from build123d import *

# Parameters (mm, degrees)
F1_DEPTH = 50
F2_R     = 8.5
F3_DEPTH = 40


with BuildPart() as f1:
    # F0 (on Top) → F1 (new body)
    with BuildSketch(Plane.XY):
        Polygon((1.650066, 3.020267), (-13.349934, 3.020267), (-13.349934, -15.979733), (1.650066, -15.979733), (7.459541, -10.479733), (7.459541, -2.479733), align=None)
    extrude(amount=F1_DEPTH)

    # F2 (on Top) → F3 (cut)
    with BuildSketch(Plane.XY):
        with Locations((-2.349934, -6.479733)):
            Circle(F2_R)
    extrude(amount=F3_DEPTH, mode=Mode.SUBTRACT)


solid = f1.part
Work out the finished part from the listing and answer in its coordinate system (mm). Round coordinates to 2 decimals unless told otherwise and drop trailing zeros. Write each loop counter-clockwise with the first axis right and the second up, starting at its lowest first coordinate (ties: lowest second). Pieces come first, ordered by that corner, then holes. Notation, with made-up numbers: M 44,-21 L 98,-21 A5 cw 98,-14 Z; hole C -20,42.5 d1. An arc over 180 degrees is marked long. Use a Markdown table: item, result.
1) Consider line 1 (Y direction, x = -2, z = 31); line 2 (Z direction, x = 4.75, y = -10.25); line 3 (X direction, y = -0.75, z = 17.5). Determine where each line is inside the solid, lowest interval first. Write a range as [from, to].
Taken from the geometry:
| item | result |
|---|---|
| line 1 | y = [-15.98, -14.97], [2.01, 3.02] |
| line 2 | z = [40, 50] |
| line 3 | x = [-13.35, -8.63], [3.93, 5.63] |
2) The part is cut by section B-B on z = 39. Give the vertices of the cut face in (x, y), plus the area to 3 significant figures.
Taken from the geometry:
| item | result |
|---|---|
| outline | M -13.35,-15.98 L 1.65,-15.98 L 7.46,-10.48 L 7.46,-2.48 L 1.65,3.02 L -13.35,3.02 Z; hole C -2.35,-6.48 d17 |
| area | 136 mm2 |
3) Flat-ended cylindrical pins translate along their axes: pin 1 (3 mm diameter, centred on x = 1, y = -7.5, fed in from -Z); pin 2 (1 mm diameter, centred on x = -10, y = -12, fed in from -Z); pin 3 (5 mm diameter, centred on x = 4.5, z = 37.5, fed in from +Y). Find the tip coordinate at first contact, or state that the pin passes through.
Taken from the geometry:
| item | result |
|---|---|
| pin 1 | stops at z = 40 |
| pin 2 | stops at z = 0 |
| pin 3 | stops at y = 2.69 |
4) The part is cut by section C-C on y = -8.5. Give the vertices of the cut face in (x, z).
Taken from the geometry:
| item | result |
|---|---|
| outline | M -13.35,0 L -10.61,0 L -10.61,40 L 5.91,40 L 5.91,0 L 7.46,0 L 7.46,50 L -13.35,50 Z |
5) The part is cut by section A-A on x = 4.25. Give the vertices of the cut face in (y, z).
Taken from the geometry:
| item | result |
|---|---|
| outline | M -13.52,0 L -11.84,0 L -11.84,40 L -1.12,40 L -1.12,0 L 0.56,0 L 0.56,50 L -13.52,50 Z |
6) Determine the mould class of faces 1 (the face through (-2, -6, 40)), 2 (the face through (-3, -6, 50)), 3 (the face through (4.6, 0.23, 24.65)), 4 (the face through (-3.456, 1.948, 19.72)) for opening direction Y: pulls with the +Y half, pulls with the -Y half, needs draft (parallel to the pull), parting line crosses it, or undercut.
Taken from the geometry:
| item | result |
|---|---|
| face 1 | undercut |
| face 2 | needs draft |
| face 3 | pulls with the +Y half |
| face 4 | undercut |
